Autodesk Inventor part; units mm, degrees
ref_plane "YZ Plane" through (0, 0, 0) normal (1, 0, 0) x (0, 1, 0)
ref_plane "XZ Plane" through (0, 0, 0) normal (0, 1, 0) x (-1, 0, 0)
ref_plane "XY Plane" through (0, 0, 0) normal (0, 0, 1) x (1, 0, 0)
sketch "草图1" plane through (0, 0, 0) normal (0, 1, 0) x (-1, 0, 0)
  line L0 (0, 65) -> (-12, 65)
  line L1 (-12, 65) -> (-12, 38)
  line L2 (-12, 38) -> (-14.5, 38)
  line L3 (-14.5, 38) -> (-14.5, 40)
  line L4 (-14.5, 40) -> (-24, 40)
  line L5 (-24, 40) -> (-24, 38)
  line L6 (-24, 38) -> (-38, 38)
  line L7 (-38, 38) -> (-38, 0)
  line L8 (-38, 0) -> (0, 0)
  line L9 (0, 0) -> (0, 65)
  line L10 (0, 38) -> (-1, 37)
  line L11 (-1, 37) -> (-1, 0)
  line L12 (-38, 34) -> (-15, 31.6998)
  line L13 (-15, 31.6998) -> (-15, 0)
  line L14 (7.6, 0) -> (-45.6, 0)
  dimension "d2" = 65
  dimension "d4" = 26
  dimension "d5" = 12
  dimension "d6" = 40
  dimension "d7" = 38
  dimension "d8" = 12
  dimension "d9" = 2.5
  dimension "d10" = 38
  dimension "d11" = 45
  dimension "d12" = 1
  dimension "d13" = 15
  dimension "d14" = 34
  dimension "d15" = 84.289
revolve "旋转1" add sketch "草图1" angle 360 about axis through (-10, 0, 0) along (1, 0, 0) contours L9 L10 L11 L8 L13 L12 L7 L6 L5 L4 L3 L2 L1 L0
sketch "草图2" plane through (0, 0, 0) normal (0, 1, 0) x (-1, 0, 0)
  line L0 (-24, 38) -> (-38, 38)
  line L1 (-38, 38) -> (-31, 38)
  line L2 (-31, 38) -> (-31, -20)
  line L3 (-31, -20) -> (-38, -20)
  line L4 (-38, -20) -> (-38, 38)
  point P0 (0, 0)
  dimension "d17" = 7
extrude "拉伸1" cut sketch "草图2" along normal mid plane 8
sketch "草图3" plane through (0, 0, 0) normal (0, 0, 1) x (1, 0, 0)
  line L0 (38, 4) -> (38, 38)
  line L1 (24, -38) -> (38, -38)
  line L2 (38, 38) -> (31, 38)
  line L3 (31, 38) -> (31, -38)
  line L4 (31, -38) -> (38, -38)
  line L5 (38, -38) -> (38, 38)
  point P0 (0, 0)
  point P1 (38, -4)
  dimension "d20" = 7
extrude "拉伸2" cut sketch "草图3" along normal mid plane 8
sketch "草图4" plane through (0, 0, 0) normal (-1, 0, 0) x (0, 0, 1)
  circle A0 centre (37.1231, 37.1231) radius 5.5
  circle A1 centre (-37.1231, 37.1231) radius 5.5
  circle A2 centre (-37.1231, -37.1231) radius 5.5
  circle A3 centre (37.1231, -37.1231) radius 5.5
  line L0 (37.1231, 37.1231) -> (0, 0)
  line L1 (0, -91) -> (0, 91)
  dimension "d23" = 11
  dimension "d24" = 52.5
  dimension "d27" = 360
  dimension "d35" = 45
extrude "拉伸3" cut sketch "草图4" against normal up to surface (12 mm away)
chamfer "倒角1" distance 1 angle 45 1 edges at (0, 0, -65)
fillet "圆角1" radius 5 1 edges at (15, 0, -31.6998)
equation "\"d2\" = 0.5 * D2"
equation "\"d4\" = M"
equation "\"d5\" = e"
equation "\"d6\" = 0.5 * D"
equation "\"d7\" = 0.5 * D_d"
equation "\"d8\" = e1"
equation "\"d10\" = 0.5 * D_d"
equation "\"d13\" = b1"
equation "\"d14\" = 0.5 * D4"
equation "\"d17\" = h_b"
equation "\"d18\" = b"
equation "\"d20\" = h_b"
equation "\"d21\" = b"
equation "\"d23\" = d0"
equation "\"d24\" = 0.5 * D0"
equation "\"d29\" = b"
equation "\"d0\" = 11"
equation "\"D0\" = 105"
equation "\"D4\" = 68"
equation "\"D_d\" = 76"
equation "\"e\" = 12"
equation "\"e1\" = 12"
equation "\"b\" = 8"
equation "\"h_b\" = 7"
equation "\"M\" = 26"
equation "\"b1\" = 15"
equation "\"d1\" = 46"
properties part number "低速轴承闷盖" material "灰口铁"
Check sheet for the modelled part. Datum: model origin and axes. Units: mm. A direction names the side the tool comes from. Coordinates: 2 decimals unless noted, no trailing zeros. Write each loop counter-clockwise with the first axis right and the second up, starting at its lowest first coordinate (ties: lowest second). Pieces come first, ordered by that corner, then holes. Notation, with made-up numbers: (60, 17) - (104, 17) arc R14 cw to (104, 26) - close; hole circle Ø10 at (-27.75, -17.75). An arc over 180 degrees is marked (long way). One line per question, with ' | ' between items.
Item 1: Sectioned sample at C-C on y = 0. Record the boundary of the cut face in (x, z), plus the area to 3 significant figures.
Determined:
outline: (0, -64) - (1, -65) - (12, -65) - (12, -38) - (14.5, -38) - (14.5, -40) - (24, -40) - (24, -38) - (38, -38) - (38, -34) - (19.5, -32.15) arc R5 cw to (15, -27.17) - (15, 27.17) arc R5 cw to (19.5, 32.15) - (31, 33.3) - (31, 38) - (24, 38) - (24, 40) - (14.5, 40) - (14.5, 38) - (12, 38) - (12, 65) - (1, 65) - (0, 64) - (0, 38) - (1, 37) - (1, -37) - (0, -38) - close | area: 1,960 mm2
Item 2: Sectioned sample at B-B on x = 3. Record the boundary of the cut face in (y, z), plus the area to 3 significant figures.
Determined:
outline: circle Ø130 at (0, 0); hole circle Ø11 at (-37.12, -37.12); hole circle Ø11 at (-37.12, 37.12); hole circle Ø11 at (37.12, -37.12); hole circle Ø11 at (37.12, 37.12) | area: 12,900 mm2
Item 3: Access from +Z, -Z, +X, -X, +Y, -Y to the whole of each face (thin tool, end or side, straight path). Record for faces 1 (the face through (1, -1, -1)), 2 (the face through (31, -35, 0)), 3 (the face through (24, 14.6, 35.4)).
Determined:
face 1: -X | face 2: +X, +Y, -Y | face 3: +X
Item 4: Mould release check, pull along Y, two halves, no side actions. Record for faces 4 (the face through (34, -35, -4)), 5 (the face through (6.58, -19.52, 62)), 6 (the face through (31, 0, 36)): pulls with the +Y half, pulls with the -Y half, needs draft (parallel to the pull), parting line crosses it, or undercut.
Determined:
face 4: needs draft | face 5: parting line crosses it | face 6: undercut
Item 5: Gauge pin test, flat ends, axial feed: P1, Ø5.5, axis at y = 35.5, z = -0.5, coming from the +X side; P2, Ø4, axis at x = 23.5, z = 17, coming from the +Y side; P3, Ø1, axis at y = 33, z = 5.5, coming from the -X side. Record the tip position at first contact, or that the pin passes through.
Determined:
P1: stops at x = 31 | P2: stops at y = 37.08 | P3: stops at x = 1
Item 6: Thickness scan on line 1 (X direction, y = 53, z = -4); line 2 (Y direction, x = 25, z = -4); line 3 (Z direction, x = 18, y = -18). Record the ranges inside material, lowest first. Write a range as [from, to].
Determined:
line 1: x = [0, 12] | line 2: y = [-37.79, -32.45], [32.45, 37.79] | line 3: z = [-35.72, -26.16], [26.16, 35.72]
Item 7: Sectioned sample at A-A on z = 0. Record the boundary of the cut face in (x, y), plus the area to 3 significant figures.
Determined:
outline: (0, -64) - (1, -65) - (12, -65) - (12, -38) - (14.5, -38) - (14.5, -40) - (24, -40) - (24, -38) - (31, -38) - (31, -33.3) - (19.5, -32.15) arc R5 cw to (15, -27.17) - (15, 27.17) arc R5 cw to (19.5, 32.15) - (31, 33.3) - (31, 38) - (24, 38) - (24, 40) - (14.5, 40) - (14.5, 38) - (12, 38) - (12, 65) - (1, 65) - (0, 64) - (0, 38) - (1, 37) - (1, -37) - (0, -38) - close | area: 1,930 mm2
